```python
from build123d import *

# Parameters (mm, degrees)
SKETCH1_R                     = 5.25
BOSS_EXTRUDE1_DEPTH           = 20
BOSS_EXTRUDE2_DEPTH           = 10
BOSS_EXTRUDE3_DEPTH           = 15
SKETCH4_R                     = 36.25
BOSS_EXTRUDE4_DEPTH           = 20
BOSS_EXTRUDE4_DRAFT           = 10
BOSS_EXTRUDE4_PROFILE_2_DEPTH = 20
BOSS_EXTRUDE4_PROFILE_2_DRAFT = 10
SKETCH5_R                     = 12.5
BOSS_EXTRUDE5_DEPTH           = 5
CUT_EXTRUDE1_DEPTH            = 196.576072156
CUT_EXTRUDE1_DEPTH_BACK       = 196.576072156
SKETCH1_2_R                   = 5.25
BOSS_EXTRUDE6_START           = 12
SKETCH6_R                     = 31
BOSS_EXTRUDE6_DEPTH           = 12
CUT_EXTRUDE2_DEPTH            = 196.576072177
CUT_EXTRUDE2_DEPTH_BACK       = 196.576072177
SKETCH3_R                     = 13.5
SKETCH3_4_R                   = 18.5
SKETCH3_4_R_2                 = 13.5
CUT_EXTRUDE3_DEPTH            = 17
SKETCH3_5_R                   = 12
CUT_EXTRUDE4_DEPTH            = 15
SKETCH3_6_R                   = 15
SKETCH3_6_R_2                 = 12
CUT_EXTRUDE5_DEPTH            = 13
SKETCH7_R                     = 17.5
CUT_EXTRUDE6_DEPTH            = 8
CUT_EXTRUDE7_DEPTH            = 198.863589399
CUT_EXTRUDE7_DEPTH_BACK       = 198.863589399
SKETCH8_R                     = 3
SKETCH9_R                     = 5.5
CUT_EXTRUDE8_DEPTH            = 6.5
SKETCH10_R                    = 12
CUT_EXTRUDE9_DEPTH            = 0.8


with BuildPart() as part:
    # Sketch1 → Boss-Extrude1 (new body)
    with BuildSketch(Plane.XY):
        with BuildLine():
            Line((-22.469211141, 130.960590801), (-122.469211141, -74.039409199))
            ThreePointArc((-122.469211141, -74.039409199), (-121.201589209, -98.247362567), (-100, -110))
            Line((-100, -110), (100, -110))
            ThreePointArc((100, -110), (121.201589209, -98.247362567), (122.469211141, -74.039409199))
            Line((122.469211141, -74.039409199), (22.469211141, 130.960590801))
            ThreePointArc((22.469211141, 130.960590801), (0, 145), (-22.469211141, 130.960590801))
        make_face()
        with Locations((0, 120)):
            Circle(SKETCH1_R, mode=Mode.SUBTRACT)
        with Locations((-100, -85)):
            Circle(SKETCH1_R, mode=Mode.SUBTRACT)
        with Locations((100, -85)):
            Circle(SKETCH1_R, mode=Mode.SUBTRACT)
    extrude(amount=BOSS_EXTRUDE1_DEPTH)

    # Sketch2 → Boss-Extrude2 (add)
    with BuildSketch(Plane.XY):
        with BuildLine():
            ThreePointArc((39.326219512, 7.310845292), (48.5, 0), (39.326219512, -7.310845292))
            ThreePointArc((39.326219512, -7.310845292), (37.73934661, -13.256761197), (35.25918145, -18.888888889))
            ThreePointArc((35.25918145, -18.888888889), (42.263103155, -63.417640882), (7.327935681, -91.902702703))
            ThreePointArc((7.327935681, -91.902702703), (0, -101), (-7.327935681, -91.902702703))
            ThreePointArc((-7.327935681, -91.902702703), (-42.263103155, -63.417640882), (-35.25918145, -18.888888889))
            ThreePointArc((-35.25918145, -18.888888889), (-37.73934661, -13.256761197), (-39.326219512, -7.310845292))
            ThreePointArc((-39.326219512, -7.310845292), (-48.5, 0), (-39.326219512, 7.310845292))
            ThreePointArc((-39.326219512, 7.310845292), (-37.73934661, 13.256761197), (-35.25918145, 18.888888889))
            ThreePointArc((-35.25918145, 18.888888889), (-42.263103155, 63.417640882), (-7.327935681, 91.902702703))
            ThreePointArc((-7.327935681, 91.902702703), (0, 101), (7.327935681, 91.902702703))
            ThreePointArc((7.327935681, 91.902702703), (42.263103155, 63.417640882), (35.25918145, 18.888888889))
            ThreePointArc((35.25918145, 18.888888889), (37.73934661, 13.256761197), (39.326219512, 7.310845292))
        make_face()
        with BuildLine():
            ThreePointArc((29.101779675, -19.444444444), (35, 0), (29.101779675, 19.444444444))
            ThreePointArc((29.101779675, 19.444444444), (0, 87.5), (-29.101779675, 19.444444444))
            ThreePointArc((-29.101779675, 19.444444444), (-35, 0), (-29.101779675, -19.444444444))
            ThreePointArc((-29.101779675, -19.444444444), (0, -87.5), (29.101779675, -19.444444444))
        make_face(mode=Mode.SUBTRACT)
    extrude(amount=-BOSS_EXTRUDE2_DEPTH)

    # Sketch2_3 → Boss-Extrude3 (add)
    with BuildSketch(Plane.XY):
        with BuildLine():
            ThreePointArc((29.101779675, 19.444444444), (0, 87.5), (-29.101779675, 19.444444444))
            ThreePointArc((-29.101779675, 19.444444444), (-35, 0), (-29.101779675, -19.444444444))
            ThreePointArc((-29.101779675, -19.444444444), (0, -87.5), (29.101779675, -19.444444444))
            ThreePointArc((29.101779675, -19.444444444), (35, 0), (29.101779675, 19.444444444))
        make_face()
        with BuildLine():
            ThreePointArc((23.778816177, 19.888888889), (0, 83.5), (-23.778816177, 19.888888889))
            ThreePointArc((-23.778816177, 19.888888889), (-31, 0), (-23.778816177, -19.888888889))
            ThreePointArc((-23.778816177, -19.888888889), (0, -83.5), (23.778816177, -19.888888889))
            ThreePointArc((23.778816177, -19.888888889), (31, 0), (23.778816177, 19.888888889))
        make_face(mode=Mode.SUBTRACT)
    extrude(amount=-BOSS_EXTRUDE3_DEPTH)


with BuildPart() as boss_extrude4_tool:
    # Sketch4 → Boss-Extrude4 (with draft: the straight prism first)
    with BuildSketch(Plane.XY.offset(20)):
        with Locations((0, 47.25)):
            Circle(SKETCH4_R)
    extrude(amount=BOSS_EXTRUDE4_DEPTH)
    # Boss-Extrude4: the draft: its side faces are tilted about the plane it starts from
    boss_extrude4_sides = [boss_extrude4_tool.faces().sort_by_distance(p)[0] for p in [
        (-36.25, 47.25, 30),
    ]]
    draft(boss_extrude4_sides, Plane.XY.offset(20), BOSS_EXTRUDE4_DRAFT)


with BuildPart() as part_1:
    add(part.part)

    # Boss-Extrude4: add boss_extrude4_tool
    add(boss_extrude4_tool.part)


with BuildPart() as boss_extrude4_profile_2_tool:
    # Sketch4 → Boss-Extrude4 profile 2 (with draft: the straight prism first)
    with BuildSketch(Plane.XY.offset(20)):
        with Locations((0, -47.25)):
            Circle(SKETCH4_R)
    extrude(amount=BOSS_EXTRUDE4_PROFILE_2_DEPTH)
    # Boss-Extrude4 profile 2: the draft: its side faces are tilted about the plane it starts from
    boss_extrude4_profile_2_sides = [boss_extrude4_profile_2_tool.faces().sort_by_distance(p)[0] for p in [
        (-36.25, -47.25, 30),
    ]]
    draft(boss_extrude4_profile_2_sides, Plane.XY.offset(20), BOSS_EXTRUDE4_PROFILE_2_DRAFT)


with BuildPart() as part_2:
    add(part_1.part)

    # Boss-Extrude4 profile 2: add boss_extrude4_profile_2_tool
    add(boss_extrude4_profile_2_tool.part)

    # Sketch5 → Boss-Extrude5 (add)
    with BuildSketch(Plane.XY.offset(20)):
        with Locations((0, 120)):
            Circle(SKETCH5_R)
        with Locations((-100, -85)):
            Circle(SKETCH5_R)
        with Locations((100, -85)):
            Circle(SKETCH5_R)
    extrude(amount=BOSS_EXTRUDE5_DEPTH)

    # Sketch1_2 → Cut-Extrude1 (cut, two sides: drawn at the far end of the back side and taken through both)
    with BuildSketch(Plane.XY.offset(-CUT_EXTRUDE1_DEPTH_BACK)):
        with Locations((0, 120)):
            Circle(SKETCH1_2_R)
        with Locations((100, -85)):
            Circle(SKETCH1_2_R)
        with Locations((-100, -85)):
            Circle(SKETCH1_2_R)
    extrude(amount=CUT_EXTRUDE1_DEPTH + CUT_EXTRUDE1_DEPTH_BACK, mode=Mode.SUBTRACT)

    # Sketch6 → Boss-Extrude6 (add)
    with BuildSketch(Plane.XY.offset(20).offset(BOSS_EXTRUDE6_START)):
        Circle(SKETCH6_R)
    extrude(amount=-BOSS_EXTRUDE6_DEPTH)

    # Sketch3 → Cut-Extrude2 (cut, two sides: drawn at the far end of the back side and taken through both)
    with BuildSketch(Plane(origin=(0, 0, 0), x_dir=(-1, 0, 0), z_dir=(0, 0, -1)).offset(-CUT_EXTRUDE2_DEPTH_BACK)):
        with Locations((0, 47.25)):
            Circle(SKETCH3_R)
        with Locations((0, -47.25)):
            Circle(SKETCH3_R)
    extrude(amount=CUT_EXTRUDE2_DEPTH + CUT_EXTRUDE2_DEPTH_BACK, mode=Mode.SUBTRACT)

    # Sketch3_4 → Cut-Extrude3 (cut)
    # profile 1 of 2: a face of its own
    with BuildSketch(Plane(origin=(0, 0, 0), x_dir=(-1, 0, 0), z_dir=(0, 0, -1))):
        with Locations((0, 47.25)):
            Circle(SKETCH3_4_R)
        with Locations((0, 47.25)):
            Circle(SKETCH3_4_R_2, mode=Mode.SUBTRACT)
    # profile 2 of 2: a face of its own
    with BuildSketch(Plane(origin=(0, 0, 0), x_dir=(-1, 0, 0), z_dir=(0, 0, -1))):
        with Locations((0, -47.25)):
            Circle(SKETCH3_4_R)
        with Locations((0, -47.25)):
            Circle(SKETCH3_4_R_2, mode=Mode.SUBTRACT)
    extrude(amount=-CUT_EXTRUDE3_DEPTH, mode=Mode.SUBTRACT)

    # Sketch3_5 → Cut-Extrude4 (cut)
    with BuildSketch(Plane(origin=(0, 0, 0), x_dir=(-1, 0, 0), z_dir=(0, 0, -1))):
        Circle(SKETCH3_5_R)
    extrude(amount=-CUT_EXTRUDE4_DEPTH, mode=Mode.SUBTRACT)

    # Sketch3_6 → Cut-Extrude5 (cut)
    with BuildSketch(Plane(origin=(0, 0, 0), x_dir=(-1, 0, 0), z_dir=(0, 0, -1))):
        Circle(SKETCH3_6_R)
        Circle(SKETCH3_6_R_2, mode=Mode.SUBTRACT)
    extrude(amount=-CUT_EXTRUDE5_DEPTH, mode=Mode.SUBTRACT)

    # Sketch7 → Cut-Extrude6 (cut)
    with BuildSketch(Plane.XY.offset(40)):
        with Locations((0, 47.25)):
            Circle(SKETCH7_R)
        with Locations((0, -47.25)):
            Circle(SKETCH7_R)
    extrude(amount=-CUT_EXTRUDE6_DEPTH, mode=Mode.SUBTRACT)

    # Sketch8 → Cut-Extrude7 (cut, two sides: drawn at the far end of the back side and taken through both)
    with BuildSketch(Plane(origin=(0, 0, -10), x_dir=(-1, 0, 0), z_dir=(0, 0, -1)).offset(-CUT_EXTRUDE7_DEPTH_BACK)):
        with Locations(Location((0, 93.5, 0), (0, 0, 180))):
            Circle(SKETCH8_R)
        with Locations(Location((41, 0, 0), (0, 0, 180))):
            Circle(SKETCH8_R)
        with Locations(Location((0, -93.5, 0), (0, 0, 180))):
            Circle(SKETCH8_R)
        with Locations(Location((-41, 0, 0), (0, 0, 180))):
            Circle(SKETCH8_R)
    extrude(amount=CUT_EXTRUDE7_DEPTH + CUT_EXTRUDE7_DEPTH_BACK, mode=Mode.SUBTRACT)

    # Sketch9 → Cut-Extrude8 (cut)
    with BuildSketch(Plane.XY.offset(20)):
        with Locations((0, 93.5)):
            Circle(SKETCH9_R)
        with Locations((-41, 0)):
            Circle(SKETCH9_R)
        with Locations((41, 0)):
            Circle(SKETCH9_R)
        with Locations((0, -93.5)):
            Circle(SKETCH9_R)
    extrude(amount=-CUT_EXTRUDE8_DEPTH, mode=Mode.SUBTRACT)

    # Sketch10 → Cut-Extrude9 (cut)
    with BuildSketch(Plane(origin=(0, 0, 0), x_dir=(-1, 0, 0), z_dir=(0, 0, -1))):
        with Locations((0, 120)):
            Circle(SKETCH10_R)
        with Locations((100, -85)):
            Circle(SKETCH10_R)
        with Locations((-100, -85)):
            Circle(SKETCH10_R)
    extrude(amount=-CUT_EXTRUDE9_DEPTH, mode=Mode.SUBTRACT)


solid = part_2.part
```
The listing builds one solid part. Answer for the finished solid, in the listing's coordinates (mm). A direction names the side the tool comes from. Coordinates: 2 decimals unless noted, no trailing zeros. Loops run counter-clockwise (first coordinate to the right, second up) from the corner with the lowest first, then second, coordinate; pieces in that order, holes last. Notation, with made-up numbers: M 89.5,-21 L 110.5,-21 A12 ccw 110.5,-14 Z; hole C -36,34.25 d7. An arc over 180 degrees is marked long. Answer as CSV lines item,"result". Start each with the question number.
(1) Given pin 1 (5.5 mm diameter, centred on x = -43.5, y = 1, fed in from +Z); pin 2 (4 mm diameter, centred on y = 61, z = 9, fed in from -X); pin 3 (5 mm diameter, centred on x = 3, y = -36.5, fed in from +Z); pin 4 (3.5 mm diameter, centred on x = -41, y = 0, fed in from -Z), each flat-ended and moving along its own axis, determine where each tip first touches the part or whether it passes through.
(2) The part is cut by section D-D (y = 120). Give the vertices of the cut face in (x, z), and give its area (3 significant figures).
(3) Find the intervals of material crossed by L1, parallel to Y at x = 41, z = -5; L2, parallel to Z at x = -20, y = -44; L3, parallel to Z at x = 85.5, y = -9, in increasing order. Write a range as [from, to].
(4) The part is cut by section B-B (z = 35.5). Give the vertices of the cut face in (x, y).
(5) The part is cut by section C-C (x = 0). State how many separate pieces and enclosed holes the cut face has, and give its area (3 significant figures).
(6) The mould has two halves that part along Y. Classify faces 1 (the flat face through (-71.769, 29.896, 9.86)), 2 (the cylindrical face through (106.72, -74.46, 22.46)), 3 (the cylindrical face through (38, 0, 2)): pulls with the +Y half, pulls with the -Y half, needs draft (parallel to the pull), parting line crosses it, or undercut.
(7) For faces 4 (the cylindrical face through (11.99, 0.53, 13.99)), 5 (the flat face through (14, -61, 40)), 6 (the cylindrical face through (-35, 0, -12)), 7 (the flat face through (73.169, 27.026, 9.86)), 8 (the cylindrical face through (-46.495, 0.242, 16.796)), determine the directions among +Z, -Z, +X, -X, +Y, -Y from which every point of the face is accessible in a straight line to the end or side of a thin tool.
Determined:
1,pin 1,"z = 13.5"
1,pin 2,"x = -57.57"
1,pin 3,"z = 32"
1,pin 4,"through"
2,outline,"M -27.82,0 L -12,0 L -12,0.8 L -5.25,0.8 L -5.25,25 L -12.5,25 L -12.5,20 L -27.82,20 Z; M 5.25,0.8 L 12,0.8 L 12,0 L 27.82,0 L 27.82,20 L 12.5,20 L 12.5,25 L 5.25,25 Z"
2,area,"964 mm2"
3,L1,"[-66.4, -28.1], [-7.5, -3], [3, 7.5], [28.1, 66.4]"
3,L2,"[0, 40]"
3,L3,"[0, 20]"
4,outline,"C 0,-47.25 d67.03; C 0,47.25 d67.03; hole C 0,-47.25 d35; hole C 0,47.25 d35"
5,separate pieces,"6"
5,enclosed holes,"0"
5,area,"4,900 mm2"
6,face 1,"pulls with the +Y half"
6,face 2,"parting line crosses it"
6,face 3,"undercut"
7,face 4,"-Z"
7,face 5,"+Z, +X, -X, +Y, -Y"
7,face 6,"-Z, -X"
7,face 7,"+Z, -Z, +X, +Y"
7,face 8,"+Z"
